```python
from build123d import *

# Parameters (mm, degrees)
F0_W     = 70
F0_H     = 70
F0_R     = 3.2
F0_R_2   = 32.25
F1_DEPTH = 31
F0_R_3   = 1.5
F2_DEPTH = 5
F3_DEPTH = 5
F5_D     = 2.4
F5_DEPTH = 8
F5_TIP   = 0.7210327428
F6_R     = 4.4


with BuildPart() as f1:
    # F0 (on Top) → F1 (new body)
    with BuildSketch(Plane.XY):
        Rectangle(F0_W, F0_H)
        with Locations((30.7, -30.7)):
            Circle(F0_R, mode=Mode.SUBTRACT)
        with Locations((-30.7, 30.7)):
            Circle(F0_R, mode=Mode.SUBTRACT)
        Circle(F0_R_2, mode=Mode.SUBTRACT)
    extrude(amount=F1_DEPTH)

    # F0 (on Top) → F2 (join)
    with BuildSketch(Plane.XY):
        with Locations((-30.7, 30.7)):
            Circle(F0_R)
        with Locations((-30.7, 30.7)):
            Circle(F0_R_3, mode=Mode.SUBTRACT)
    extrude(amount=F2_DEPTH)

    # F0 (on Top) → F3 (join)
    with BuildSketch(Plane.XY):
        with Locations((30.7, -30.7)):
            Circle(F0_R)
        with Locations((30.7, -30.7)):
            Circle(F0_R_3, mode=Mode.SUBTRACT)
    extrude(amount=F3_DEPTH)

    # F5
    with Locations(Plane.XY.offset(31)):
        with Locations((-25, -25), (25, 25), (-25, 25), (25, -25)):
            Hole(F5_D / 2, depth=F5_DEPTH)
            with Locations((0, 0, -(F5_DEPTH + F5_TIP / 2))):  # 118° drill point
                Cone(0, F5_D / 2, F5_TIP, mode=Mode.SUBTRACT)

    # F6
    f6_edges = [f1.edges().sort_by_distance(p)[0] for p in [
        (-35, -35, 15.5),
        (35, -35, 15.5),
        (35, 35, 15.5),
        (-35, 35, 15.5),
    ]]
    fillet(f6_edges, radius=F6_R)


solid = f1.part
```
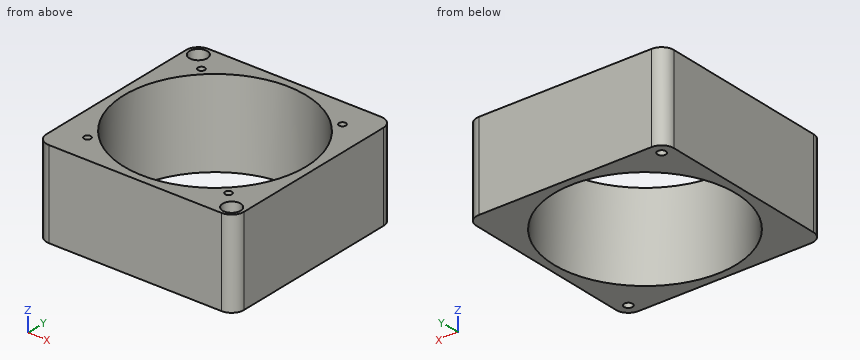
Work out the finished part from the listing and answer in its coordinate system (mm). Give positions to 0.01 mm unless a question says otherwise; leave off trailing zeros. Write each loop counter-clockwise with the first axis right and the second up, starting at its lowest first coordinate (ties: lowest second). Pieces come first, ordered by that corner, then holes. Notation, with made-up numbers: (4, 48.25) -> (51, 48.25) arc R10 cw to (51, 59.25) -> close; hole circle Ø4 at (-36, 82). An arc over 180 degrees is marked (long way). Write item = value, one per line.
Q1. Section D-D on z = 19 is taken. Determine the outline of the cut face in (x, y), and give its area (3 significant figures).
Computed values:
outline = (-35, -30.6) arc R4.4 ccw to (-30.6, -35) -> (30.6, -35) arc R4.4 ccw to (35, -30.6) -> (35, 30.6) arc R4.4 ccw to (30.6, 35) -> (-30.6, 35) arc R4.4 ccw to (-35, 30.6) -> close; hole circle Ø6.4 at (-30.7, 30.7); hole circle Ø64.5 at (0, 0); hole circle Ø6.4 at (30.7, -30.7)
area = 1,550 mm^2
Q2. Section B-B on x = 0 is taken. Determine the outline of the cut face in (y, z), and give its area (4 significant figures).
Computed values:
outline = (-35, 0) -> (-32.25, 0) -> (-32.25, 31) -> (-35, 31) -> close; (32.25, 0) -> (35, 0) -> (35, 31) -> (32.25, 31) -> close
area = 170.5 mm^2
Q3. Flat-ended cylindrical pins translate along their axes: pin 1 Ø2.5 at (x, y) = (30.7, -30.7) entering from -Z; pin 2 Ø6 at (x, y) = (30.7, -30.7) entering from +Z; pin 3 Ø1.4 at (x, y) = (25, -25) entering from +Z. Find the tip coordinate at first contact, or state that the pin passes through.
Computed values:
pin_1 = through
pin_2 = 5
pin_3 = 22.7
Q4. Consider line 1 along Y through (x, z) = (1, 17); line 2 along Y through (x, z) = (25, 28.75); line 3 along X through (y, z) = (25, 19). Determine where each line is inside the solid, lowest interval first.
Computed values:
line_1 = -35 to -32.23, 32.23 to 35
line_2 = -35 to -26.2, -23.8 to -20.37, 20.37 to 23.8, 26.2 to 35
line_3 = -35 to -20.37, 20.37 to 35
Q5. Section A-A on z = 29 is taken. Determine the outline of the cut face in (x, y), and give its area (3 significant figures).
Computed values:
outline = (-35, -30.6) arc R4.4 ccw to (-30.6, -35) -> (30.6, -35) arc R4.4 ccw to (35, -30.6) -> (35, 30.6) arc R4.4 ccw to (30.6, 35) -> (-30.6, 35) arc R4.4 ccw to (-35, 30.6) -> close; hole circle Ø6.4 at (-30.7, 30.7); hole circle Ø64.5 at (0, 0); hole circle Ø2.4 at (-25, -25); hole circle Ø2.4 at (-25, 25); hole circle Ø2.4 at (25, -25); hole circle Ø2.4 at (25, 25); hole circle Ø6.4 at (30.7, -30.7)
area = 1,530 mm^2
